Geometry: final body of the model. Coordinates: model frame, mm. A direction names the side the tool comes from. Give positions to 0.01 mm unless a question says otherwise; leave off trailing zeros. Write each loop counter-clockwise with the first axis right and the second up, starting at its lowest first coordinate (ties: lowest second). Pieces come first, ordered by that corner, then holes. Notation, with made-up numbers: (-17, 53) -> (-8, 53) arc R20 ccw to (-8, 86) -> close; hole circle Ø3 at (16.5, 72). An arc over 180 degrees is marked (long way). Answer in a Markdown table with one row per item. Add a question column.
from build123d import *

# Parameters (mm, degrees)
BOSS_EXTRUDE1_DEPTH = 76.2
SKETCH7_R           = 2.4892
CUT_EXTRUDE4_DEPTH  = 84.339970152
SKETCH8_R           = 2.4892
CUT_EXTRUDE5_DEPTH  = 84.339970152


with BuildPart() as part:
    # Sketch1 → Boss-Extrude1 (new body)
    with BuildSketch(Plane.XY):
        Polygon((3.175, 25.4), (3.175, 3.175), (25.4, 3.175), (25.4, 0), (0, 0), (0, 25.4), align=None)
    extrude(amount=BOSS_EXTRUDE1_DEPTH)

    # Sketch7 → Cut-Extrude4 (cut, through all)
    with BuildSketch(Plane(origin=(3.175, 0, 0), x_dir=(0, 0, -1), z_dir=(1, 0, 0))):
        with Locations(Location((-63.5, 12.7, 0), (0, 0, 90))):
            Circle(SKETCH7_R)
        with Locations(Location((-38.1, 12.7, 0), (0, 0, 90))):
            Circle(SKETCH7_R)
        with Locations(Location((-12.7, 12.7, 0), (0, 0, 90))):
            Circle(SKETCH7_R)
    extrude(amount=-CUT_EXTRUDE4_DEPTH, mode=Mode.SUBTRACT)

    # Sketch8 → Cut-Extrude5 (cut, through all)
    with BuildSketch(Plane(origin=(0, 3.175, 0), x_dir=(1, 0, 0), z_dir=(0, 1, 0))):
        with Locations(Location((12.7, -38.1, 0), (0, 0, 270))):
            Circle(SKETCH8_R)
    extrude(amount=-CUT_EXTRUDE5_DEPTH, mode=Mode.SUBTRACT)


solid = part.part
Q1. Pull-direction query (Z, two-part tool) for faces 3 (the flat face through (7, 2, 0)), 4 (the flat face through (2, 25.4, 38)), 5 (the cylindrical face through (1.61, 12.16, 35.67)), 6 (the flat face through (7, 2, 76.2)); classes: +Z half, -Z half, draft (parallel to the pull), parting line (faces both ways), or undercut.
Q2. Access query for faces 1 (the flat face through (17, 3.175, 38)), 2 (the flat face through (25.4, 2, 38)). Directions: +Z, -Z, +X, -X, +Y, -Y. A direction counts if a zero-diameter tool reaches every point of the face in a straight line with its end or side. Return the directions, or none.
Q3. Section B-B on x = 12.7. Return loops of the section in (y, z) (3 decimals).
Q4. Section D-D on z = 38.1. Return loops of the section in (x, y) (3 decimals).
Q5. Section A-A on z = 63.5. Return loops of the section in (x, y) (3 decimals), and give its area (3 significant figures).
Q6. Line query: probe 1 along Z at (x, y) = (1.9, 12.7); probe 2 along Y at (x, z) = (11.75, 40.5) (3 decimals). Output: solid intervals per line, ascending. Write a range as from..to.
Q7. Contact query for flat-ended pins moving along their axis: pin 1 Ø6.5 at (y, z) = (12.7, 12.7) entering from +X (3 decimals); pin 2 Ø6 at (x, z) = (23, 63.5) entering from +Y (3 decimals). Output: stop coordinate, or through.
Q8. Section C-C on y = 12.7. Return loops of the section in (x, z) (3 decimals).
Checks:
| question | item | result |
|---|---|---|
| 1 | face 3 | -Z half |
| 1 | face 4 | draft |
| 1 | face 5 | undercut |
| 1 | face 6 | +Z half |
| 2 | face 1 | +Z, -Z, +X, +Y |
| 2 | face 2 | +Z, -Z, +X, +Y, -Y |
| 3 | outline | (0, 0) -> (3.175, 0) -> (3.175, 35.611) -> (0, 35.611) -> close; (0, 40.589) -> (3.175, 40.589) -> (3.175, 76.2) -> (0, 76.2) -> close |
| 4 | outline | (0, 0) -> (10.211, 0) -> (10.211, 3.175) -> (3.175, 3.175) -> (3.175, 10.211) -> (0, 10.211) -> close; (0, 15.189) -> (3.175, 15.189) -> (3.175, 25.4) -> (0, 25.4) -> close; (15.189, 0) -> (25.4, 0) -> (25.4, 3.175) -> (15.189, 3.175) -> close |
| 5 | outline | (0, 0) -> (25.4, 0) -> (25.4, 3.175) -> (3.175, 3.175) -> (3.175, 10.211) -> (0, 10.211) -> close; (0, 15.189) -> (3.175, 15.189) -> (3.175, 25.4) -> (0, 25.4) -> close |
| 5 | area | 135 mm^2 |
| 6 | probe 1 | 0..10.21, 15.19..35.61, 40.59..61.01, 65.99..76.2 |
| 6 | probe 2 | 0..3.175 |
| 7 | pin 1 | x = 3.175 |
| 7 | pin 2 | y = 3.175 |
| 8 | outline | (0, 0) -> (3.175, 0) -> (3.175, 10.211) -> (0, 10.211) -> close; (0, 15.189) -> (3.175, 15.189) -> (3.175, 35.611) -> (0, 35.611) -> close; (0, 40.589) -> (3.175, 40.589) -> (3.175, 61.011) -> (0, 61.011) -> close; (0, 65.989) -> (3.175, 65.989) -> (3.175, 76.2) -> (0, 76.2) -> close |
